```python
from build123d import *

# Parameters (mm, degrees)
F0_R     = 15.875
F1_DEPTH = 25.4
F2_DEPTH = 25.4


with BuildPart() as f1:
    # F0 (on Front) → F1 (new body)
    with BuildSketch(Plane.XZ):
        with BuildLine():
            ThreePointArc((13.163634, -28.892581), (26.702134, -17.177269), (31.75, 0))
            ThreePointArc((31.75, 0), (25.188056, 19.329365), (8.214608, 30.668921))
            ThreePointArc((8.214608, 30.668921), (-31.640961, -2.62908), (13.163634, -28.892581))
        make_face()
        with BuildLine():
            ThreePointArc((-15.143785, 4.7625), (0, 15.875), (15.143785, 4.7625))
            Line((15.143785, 4.7625), (19.05, 4.7625))
            Line((19.05, 4.7625), (19.05, -4.7625))
            Line((19.05, -4.7625), (15.143785, -4.7625))
            ThreePointArc((15.143785, -4.7625), (0, -15.875), (-15.143785, -4.7625))
            Line((-15.143785, -4.7625), (-19.05, -4.7625))
            Line((-19.05, -4.7625), (-19.05, 4.7625))
            Line((-19.05, 4.7625), (-15.143785, 4.7625))
        make_face(mode=Mode.SUBTRACT)
        with BuildLine():
            ThreePointArc((73.025, 0), (66.721746, 14.157082), (51.983218, 18.945588))
            ThreePointArc((51.983218, 18.945588), (34.956217, -1.090134), (54.161027, -19.049092))
            ThreePointArc((54.161027, -19.049092), (67.510995, -13.404452), (73.025, 0))
        make_face()
        with Locations((53.975, 0)):
            Circle(F0_R, mode=Mode.SUBTRACT)
        with BuildLine():
            ThreePointArc((8.214608, 30.668921), (25.188056, 19.329365), (31.75, 0))
            ThreePointArc((31.75, 0), (26.702134, -17.177269), (13.163634, -28.892581))
            Line((13.163634, -28.892581), (54.161027, -19.049092))
            ThreePointArc((54.161027, -19.049092), (34.956217, -1.090134), (51.983218, 18.945588))
            Line((51.983218, 18.945588), (8.214608, 30.668921))
        make_face()
        with BuildLine():
            ThreePointArc((-15.143785, -4.7625), (-15.875, 0), (-15.143785, 4.7625))
            Line((-15.143785, 4.7625), (-19.05, 4.7625))
            Line((-19.05, 4.7625), (-19.05, -4.7625))
            Line((-19.05, -4.7625), (-15.143785, -4.7625))
        make_face()
    extrude(amount=F1_DEPTH)

    # F0 (on Front) → F2 (join)
    with BuildSketch(Plane.XZ):
        with BuildLine():
            ThreePointArc((13.163634, -28.892581), (26.702134, -17.177269), (31.75, 0))
            ThreePointArc((31.75, 0), (25.188056, 19.329365), (8.214608, 30.668921))
            ThreePointArc((8.214608, 30.668921), (-31.640961, -2.62908), (13.163634, -28.892581))
        make_face()
        with BuildLine():
            ThreePointArc((-15.143785, 4.7625), (0, 15.875), (15.143785, 4.7625))
            Line((15.143785, 4.7625), (19.05, 4.7625))
            Line((19.05, 4.7625), (19.05, -4.7625))
            Line((19.05, -4.7625), (15.143785, -4.7625))
            ThreePointArc((15.143785, -4.7625), (0, -15.875), (-15.143785, -4.7625))
            Line((-15.143785, -4.7625), (-19.05, -4.7625))
            Line((-19.05, -4.7625), (-19.05, 4.7625))
            Line((-19.05, 4.7625), (-15.143785, 4.7625))
        make_face(mode=Mode.SUBTRACT)
        with BuildLine():
            ThreePointArc((-15.143785, -4.7625), (-15.875, 0), (-15.143785, 4.7625))
            Line((-15.143785, 4.7625), (-19.05, 4.7625))
            Line((-19.05, 4.7625), (-19.05, -4.7625))
            Line((-19.05, -4.7625), (-15.143785, -4.7625))
        make_face()
    extrude(amount=-F2_DEPTH)


solid = f1.part
```
Part model, mm, in its own coordinate system. A direction names the side the tool comes from. Round coordinates to 2 decimals unless told otherwise and drop trailing zeros. Write each loop counter-clockwise with the first axis right and the second up, starting at its lowest first coordinate (ties: lowest second). Pieces come first, ordered by that corner, then holes. Notation, with made-up numbers: (80, 75) -> (103, 75) arc R28 cw to (103, 103) -> close; hole circle Ø5 at (8.5, 17). An arc over 180 degrees is marked (long way). Return JSON: item names as keys, results as strings. Group by question number.
Q1. Saw through at D-D on y = -2. State how many separate pieces and enclosed holes the cut face has, plus the area to 3 significant figures.
Q2. Mould opens along Z. For faces 4 (the cylindrical face through (69.117, -12.522, 4.768)), 5 (the flat face through (33.38, -12.52, -24.04)), 6 (the flat face through (30.405, -12.522, 24.725)), 7 (the flat face through (17, 0, -4.762)) say: pulls with the +Z half, pulls with the -Z half, needs draft (parallel to the pull), parting line crosses it, or undercut.
Q3. Saw through at C-C on z = 1.5. Write the cut outline in (x, y), plus the area to 3 significant figures.
Q4. Saw through at A-A on x = 0. Write the cut outline in (y, z) (3 decimals), plus the area to 3 significant figures.
Q5. Which spindle directions (+Z, -Z, +X, -X, +Y, -Y) get a long thin tool onto all of the face, cutting with end or side? Do faces 1 (the flat face through (-15, 25.4, -7)), 2 (the flat face through (17, 0, 4.762)), 3 (the flat face through (38, 0, 3)). Say none if no direction does.
Q6. Pin check, flat tips, straight feed: pin 1 (2 mm diameter, centred on x = 17.5, y = 8, fed in from -Z); pin 2 (6 mm diameter, centred on y = 7, z = 1, fed in from +X); pin 3 (1.5 mm diameter, centred on y = 1.5, z = 1, fed in from -X); pin 4 (4 mm diameter, centred on y = -13.5, z = -14.5, fed in from +X). Stop position of each tip, or through.
Q7. Probe L1, parallel to Y at x = 44.5, z = 15.5; L2, parallel to Z at x = -9, y = 3; L3, parallel to Z at x = 16, y = -13.5. List the from-to ranges inside material, lowest first. Write a range as [from, to].
Answer:
{
 "1": {"separate pieces": "1", "enclosed holes": "2", "area": "3,300 mm2"},
 "2": {"face 4": "undercut", "face 5": "pulls with the -Z half", "face 6": "pulls with the +Z half", "face 7": "undercut"},
 "3": {"outline": "(-31.71, -25.4) -> (-15.8, -25.4) -> (-15.8, 25.4) -> (-31.71, 25.4) -> close; (19.05, -25.4) -> (38.17, -25.4) -> (38.17, 0) -> (31.71, 0) -> (31.71, 25.4) -> (19.05, 25.4) -> close; (69.78, -25.4) -> (72.97, -25.4) -> (72.97, 0) -> (69.78, 0) -> close", "area": "1,700 mm2"},
 "4": {"outline": "(-25.4, -31.75) -> (25.4, -31.75) -> (25.4, -15.875) -> (-25.4, -15.875) -> close; (-25.4, 15.875) -> (25.4, 15.875) -> (25.4, 31.75) -> (-25.4, 31.75) -> close", "area": "1,610 mm2"},
 "5": {"face 1": "+Z, -Z, +X, -X, +Y", "face 2": "+Y, -Y", "face 3": "+X, +Y"},
 "6": {"pin 1": "z = -27.13", "pin 2": "x = 31.75", "pin 3": "x = -31.75", "pin 4": "x = 68.35"},
 "7": {"L1": "[-25.4, 0]", "L2": "[-30.45, -13.08], [13.08, 30.45]", "L3": "[-28.21, -4.76], [4.76, 28.58]"}
}
